```python
from build123d import *

# Parameters (mm, degrees)
F1_DEPTH  = 31.75
F2_W      = 139.7
F2_H      = 152.4
F3_DEPTH  = 25.4
F5_D      = 31.75
F6_W      = 31.75
F6_H      = 31.75
F6_H_2    = 88.9
F7_DEPTH  = 19.05
F8_W      = 31.75
F8_H      = 31.75
F9_DEPTH  = 19.05
F10_W     = 31.75
F10_H     = 31.75
F11_DEPTH = 19.05


with BuildPart() as f1:
    # F0 (on Top) → F1 (new body)
    with BuildSketch(Plane.XY):
        Polygon((154.9607325792, 50.8), (-99.0392674208, 50.8), (-99.0392674208, 0), (-57.7642674208, 0), (-57.7642674208, -50.8), (-99.0392674208, -50.8), (-99.0392674208, -101.6), (154.9607325792, -101.6), (154.9607325792, -50.8), (113.6857325792, -50.8), (113.6857325792, 0), (154.9607325792, 0), align=None)
    extrude(amount=F1_DEPTH)

    # F2 (on face) → F3 (join)
    with BuildSketch(Plane.XY.offset(31.75)):
        with Locations((27.9607325792, -25.4)):
            Rectangle(F2_W, F2_H)
    extrude(amount=F3_DEPTH)

    # F5 (through all)
    with Locations(Plane.XY.offset(57.15)):
        with Locations((23.8818004727, -15.8603843302)):
            Hole(F5_D / 2)

    # F6 (on face) → F7 (join)
    with BuildSketch(Plane.XY.offset(57.15)):
        with Locations((-26.0142674208, -85.725)):
            Rectangle(F6_W, F6_H)
        with Locations((-26.0142674208, 34.925)):
            Rectangle(F6_W, F6_H)
        with Locations((81.9357325792, 34.925)):
            Rectangle(F6_W, F6_H)
        with Locations((81.9357325792, -85.725)):
            Rectangle(F6_W, F6_H)
        with Locations((-26.0142674208, -25.4)):
            Rectangle(F6_W, F6_H_2)
        with Locations((81.9357325792, -25.4)):
            Rectangle(F6_W, F6_H_2)
    extrude(amount=F7_DEPTH)

    # F8 (on face) → F9 (join)
    with BuildSketch(Plane.XY.offset(76.2)):
        with Locations((-26.0142674208, -85.725)):
            Rectangle(F8_W, F8_H)
        with Locations((-26.0142674208, 34.925)):
            Rectangle(F8_W, F8_H)
    extrude(amount=F9_DEPTH)

    # F10 (on face) → F11 (join)
    with BuildSketch(Plane.XY.offset(76.2)):
        with Locations((81.9357325792, -85.725)):
            Rectangle(F10_W, F10_H)
        with Locations((81.9357325792, 34.925)):
            Rectangle(F10_W, F10_H)
    extrude(amount=F11_DEPTH)


solid = f1.part
```
Could you check a few things on this model? Use its own coordinates, in mm. A direction names the side the tool comes from. Coordinates: 2 decimals unless noted, no trailing zeros. Write each loop counter-clockwise with the first axis right and the second up, starting at its lowest first coordinate (ties: lowest second). Pieces come first, ordered by that corner, then holes. Notation, with made-up numbers: (66.5, -5) -> (93.5, -5) arc R25 cw to (93.5, 18) -> close; hole circle Ø9 at (3.5, 17). An arc over 180 degrees is marked (long way). One line per question, with ' | ' between items. Start each with the question number.
1. If we section it at A-A (x = 137.5): Please give me the cut outline in (y, z).
2. If we section it at B-B (z = 66.5): Please give me the cut outline in (x, y), and give its area (3 significant figures).
3. If we section it at D-D (x = 73.5): Please give me the cut outline in (y, z).
4. Thinking about a two-plate mould opening in Y: for faces 1 (the face through (26, -101.6, 36)), 2 (the face through (154.961, -77, 16)), 3 (the face through (82, 19.05, 86)), which applies, pulls with the +Y half, pulls with the -Y half, needs draft (parallel to the pull), parting line crosses it, or undercut?
5. If we section it at C-C (y = -18.5): Please give me the cut outline in (x, z), and give its area (3 significant figures).
6. Please list where these lines run through material, in increasing order: line 1 along Y through (x, z) = (93, 82.5); line 2 along X through (y, z) = (32, 60); line 3 along Y through (x, z) = (-78.5, 8.5).
7. Will these pins go through, and if not, where does the flat tip stop? P1, Ø4, axis at y = -45.5, z = 63.5, coming from the +X side; P2, Ø2, axis at x = 80, y = -39, coming from the +Z side.
8. For faces 4 (the face through (134, 0, 16)), 5 (the face through (-26, -25, 76.2)), 6 (the face through (97.811, -26, 56)), 7 (the face through (-41.889, -26, 56)), 8 (the face through (-10.139, -26, 72)), which set-ups out of +Z, -Z, +X, -X, +Y, -Y let a thin tool reach every point of the face, with its end or its side?
Return value:
1) outline: (-101.6, 0) -> (-50.8, 0) -> (-50.8, 31.75) -> (-101.6, 31.75) -> close; (0, 0) -> (50.8, 0) -> (50.8, 31.75) -> (0, 31.75) -> close
2) outline: (-41.89, -101.6) -> (-10.14, -101.6) -> (-10.14, 50.8) -> (-41.89, 50.8) -> close; (66.06, -101.6) -> (97.81, -101.6) -> (97.81, 50.8) -> (66.06, 50.8) -> close | area: 9,680 mm²
3) outline: (-101.6, 0) -> (50.8, 0) -> (50.8, 95.25) -> (19.05, 95.25) -> (19.05, 76.2) -> (-69.85, 76.2) -> (-69.85, 95.25) -> (-101.6, 95.25) -> close
4) face 1: pulls with the -Y half | face 2: needs draft | face 3: undercut
5) outline: (-57.76, 0) -> (8.23, 0) -> (8.23, 57.15) -> (-10.14, 57.15) -> (-10.14, 76.2) -> (-41.89, 76.2) -> (-41.89, 31.75) -> (-57.76, 31.75) -> close; (39.54, 0) -> (113.69, 0) -> (113.69, 31.75) -> (97.81, 31.75) -> (97.81, 76.2) -> (66.06, 76.2) -> (66.06, 57.15) -> (39.54, 57.15) -> close | area: 8,410 mm²
6) line 1: y = -101.6 to -69.85, 19.05 to 50.8 | line 2: x = -41.89 to -10.14, 66.06 to 97.81 | line 3: y = -101.6 to -50.8, 0 to 50.8
7) P1: stops at x = 97.81 | P2: stops at z = 76.2
8) face 4: +Z, -Z, +X | face 5: +Z, +X, -X | face 6: +Z, +X, +Y, -Y | face 7: +Z, -X, +Y, -Y | face 8: +Z, +Y, -Y
